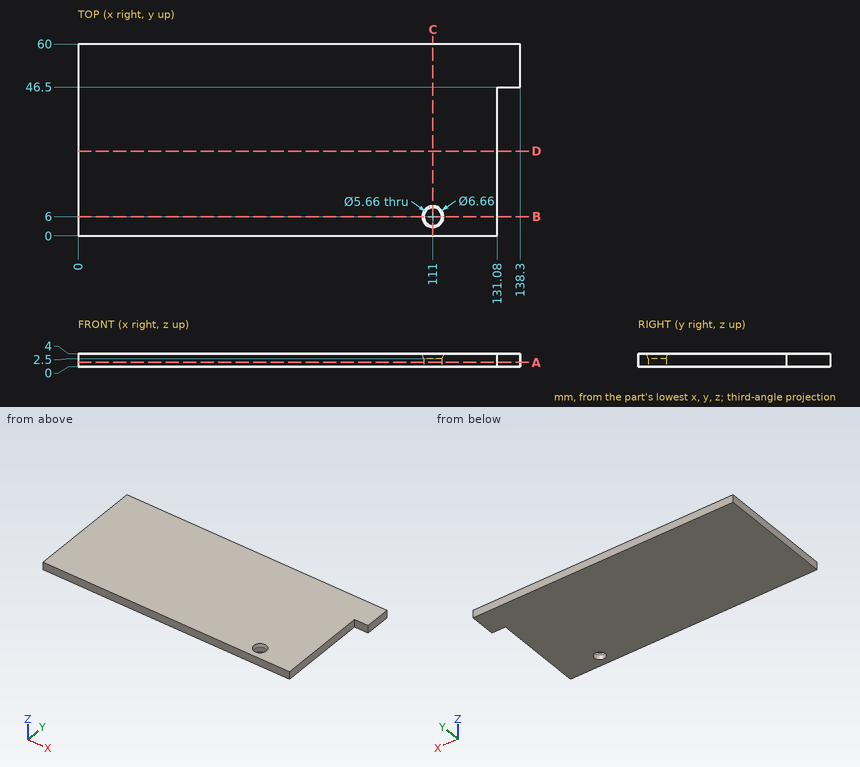
Can you work these out from the drawing? Everything is in mm from the part's minimum corner. Give positions to 0.01 mm unless a question says otherwise; leave off trailing zeros. Order: outer loops, then holes, each group sorted by start corner. A loop starts at its lowest first (then second) coordinate and runs counter-clockwise, first axis right, second up. Notation, with made-up numbers: M -21.75,33 L 28.25,33 A16 ccw 28.25,45 Z; hole C 1.25,69 d3. An arc over 180 degrees is marked long. Use a Markdown table: item, result. Add a question column.
1. Suppose I cut it at D-D (y = 26.5). List the corners of the cut face in (x, z) for me, and give its area (3 significant figures).
2. Suppose I cut it at B-B (y = 6). List the corners of the cut face in (x, z) for me.
3. For pin 1 Ø1 at (y, z) = (38.5, 0.5) entering from +X; pin 2 Ø3.5 at (x, y) = (111, 6) entering from +Z, each with a flat end and sliding along its axis, tell me the tip position at first contact or that it passes through.
4. Suppose I cut it at A-A (z = 1.35). List the corners of the cut face in (x, y) for me.
5. Suppose I cut it at C-C (x = 111). List the corners of the cut face in (y, z) for me, and give its area (3 significant figures).
6. I need wall thicknesses on probe 1 along Y at (x, z) = (111, 0.6); probe 2 along X at (y, z) = (39.5, 3.3); probe 3 along X at (y, z) = (5, 3.2) (1 decimal). Which ranges of each line are inside material? Lowest first, please. Write a range as from..to.
Results list:
| question | item | result |
|---|---|---|
| 1 | outline | M 0,0 L 131.08,0 L 131.08,4 L 0,4 Z |
| 1 | area | 524 mm² |
| 2 | outline | M 0,0 L 108.17,0 L 108.17,2.5 L 107.67,4 L 0,4 Z; M 113.83,0 L 131.08,0 L 131.08,4 L 114.33,4 L 113.83,2.5 Z |
| 3 | pin 1 | stops at x = 131.08 |
| 3 | pin 2 | passes through |
| 4 | outline | M 0,0 L 131.08,0 L 131.08,46.5 L 138.3,46.5 L 138.3,60 L 0,60 Z; hole C 111,6 d5.66 |
| 5 | outline | M 0,0 L 3.17,0 L 3.17,2.5 L 2.67,4 L 0,4 Z; M 8.83,0 L 60,0 L 60,4 L 9.33,4 L 8.83,2.5 Z |
| 5 | area | 217 mm² |
| 6 | probe 1 | y = 0..3.17, 8.83..60 |
| 6 | probe 2 | x = 0..131.08 |
| 6 | probe 3 | x = 0..108.1, 113.9..131.1 |
